Study the drawing (mm; zero at the part's minimum x, y, z) and answer. A direction names the side the tool comes from. Give positions to 0.01 mm unless a question says otherwise; leave off trailing zeros. Loops run counter-clockwise (first coordinate to the right, second up) from the corner with the lowest first, then second, coordinate; pieces in that order, holes last. Notation, with made-up numbers: (-30, -25.5) -> (-25, -25.5) arc R24 cw to (-25, 1.5) -> close; hole circle Ø10 at (48.5, -14). An arc over 180 degrees is marked (long way). One line per question, with ' | ' between items. Start each with the question number.
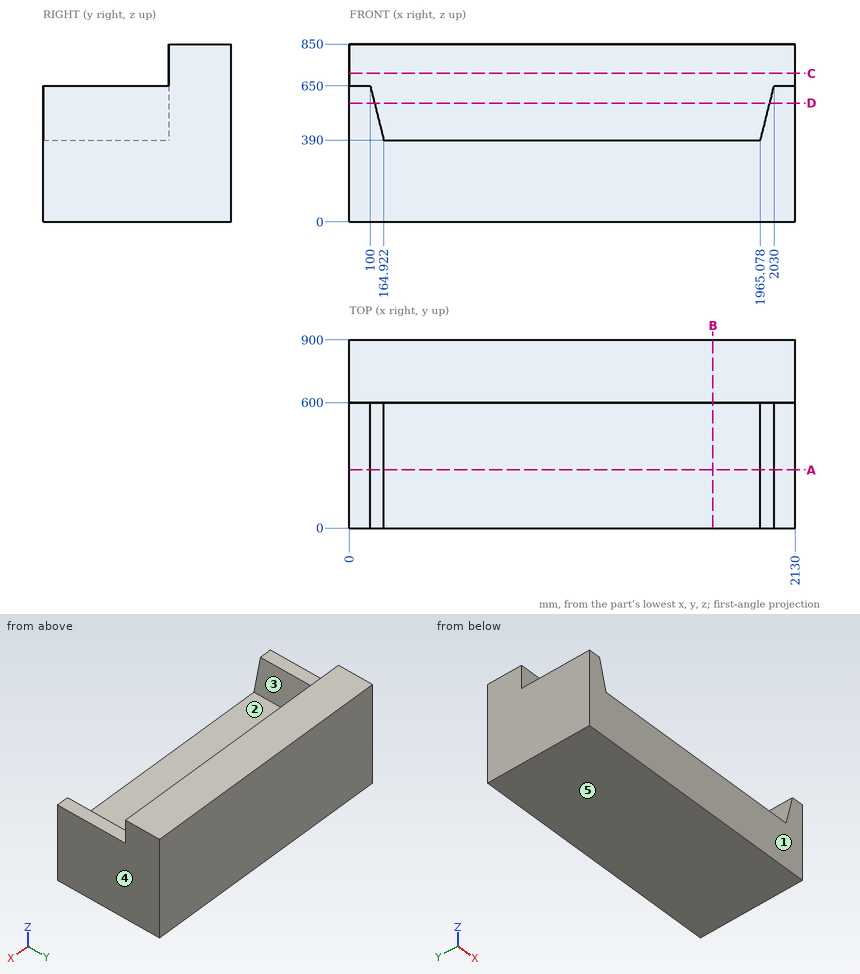
1. The part is cut by section C-C (z = 710). Write down the section's boundary in (x, y).
2. The part is cut by section D-D (z = 568). Write down the section's boundary in (x, y) (1 decimal).
3. For the marked faces 1 and 2, determine the directions among +Z, -Z, +X, -X, +Y, -Y from which every point of the face is accessible in a straight line to the end or side of a thin tool.
4. Straight lines are drawn through the part: L1, parallel to Z at x = 1446.5, y = 509.5; L2, parallel to X at y = 310.5, z = 431; L3, parallel to Y at x = 1043, z = 528. For each, find the intervals that lie inside material, in ascending order.
5. The part is cut by section A-A (y = 279). Write down the section's boundary in (x, z).
6. The part is cut by section B-B (x = 1737). Write down the section's boundary in (y, z).
7. Determine the mould class of the marked faces 3, 4 and 5 for opening direction X: released by +X, released by -X, zero draft, split by the parting line, or undercut.
8. This flat-tipped pin is pushed along its axis until it touches: pin 1 Ø12 at (x, y) = (1649.5, 422) entering from +Z. Where does it stop, or does it pass through?
Check sheet entries:
1) outline: (0, 600) -> (2130, 600) -> (2130, 900) -> (0, 900) -> close
2) outline: (0, 0) -> (120.5, 0) -> (120.5, 600) -> (2009.5, 600) -> (2009.5, 0) -> (2130, 0) -> (2130, 900) -> (0, 900) -> close
3) face 1: +Z, -Z, +X, -X, -Y | face 2: +Z, -Y
4) L1: z = 0 to 390 | L2: x = 0 to 154.68, 1975.32 to 2130 | L3: y = 600 to 900
5) outline: (0, 0) -> (2130, 0) -> (2130, 650) -> (2030, 650) -> (1965.08, 390) -> (164.92, 390) -> (100, 650) -> (0, 650) -> close
6) outline: (0, 0) -> (900, 0) -> (900, 850) -> (600, 850) -> (600, 390) -> (0, 390) -> close
7) face 3: undercut | face 4: released by +X | face 5: zero draft
8) pin 1: stops at z = 390
